Verification items for the finished model (mm, model axes). Round coordinates to 2 decimals unless told otherwise and drop trailing zeros. Order: outer loops, then holes, each group sorted by start corner. A loop starts at its lowest first (then second) coordinate and runs counter-clockwise, first axis right, second up. Notation, with made-up numbers: M 76.5,-8.5 L 121.5,-8.5 A17 cw 121.5,6.5 Z; hole C 83.5,50.25 d2. An arc over 180 degrees is marked long. Use one line per item in the form item = value. Start each with the question number.
Item 1: Cross-section at A-A on x = -7. Enter the section's corners in (y, z).
Item 2: Go/stop test with flat-tipped pins: pin 1 Ø0.6 at (x, z) = (-41, 1.5) entering from +Y; pin 2 Ø1 at (y, z) = (-16.5, 1) entering from -X. Record where each tip stops, or that it passes through.
Item 3: Thickness scan on probe 1 along X at (y, z) = (-7.75, 1.2); probe 2 along X at (y, z) = (-10.25, 1.7); probe 3 along Y at (x, z) = (-41, 1.05). Record the ranges inside material, lowest first. Write a range as [from, to].
Item 4: Cross-section at B-B on x = -35. Enter the section's corners in (y, z).
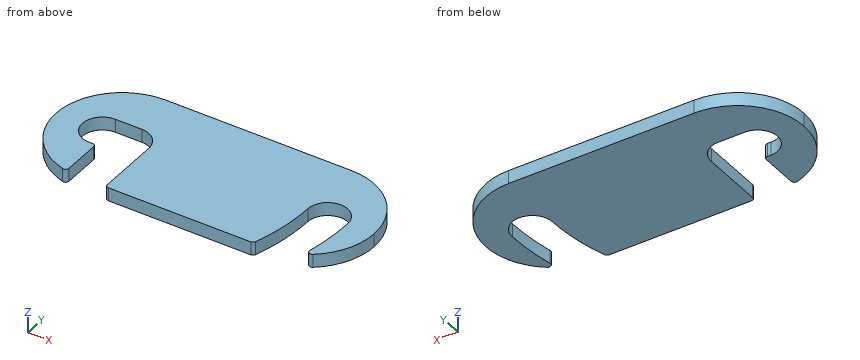
from build123d import *

# Parameters (mm, degrees)
SZKIC1_W                    = 48
SZKIC1_H                    = 20
SZKIC1_R                    = 3
DODANIE_WYCI_GNI_CIE2_DEPTH = 2
ZAOKR_GLENIE3_R             = 10
WYTNIJ_WYCI_GNI_CIE1_DEPTH  = 53.038447325
ZAOKR_GLENIE1_R             = 3
ZAOKR_GLENIE2_R             = 0.5


with BuildPart() as part:
    # Szkic1 → Dodanie-wyciągnięcie2 (new body)
    with BuildSketch(Plane.XY):
        with Locations((-24, -10)):
            Rectangle(SZKIC1_W, SZKIC1_H)
        with Locations((-7, -10)):
            Circle(SZKIC1_R, mode=Mode.SUBTRACT)
        with Locations((-41, -10)):
            Circle(SZKIC1_R, mode=Mode.SUBTRACT)
    extrude(amount=DODANIE_WYCI_GNI_CIE2_DEPTH)

    # Zaokrąglenie3
    zaokr_glenie3_edges = [part.edges().sort_by_distance(p)[0] for p in [
        (0, 0, 1),
        (0, -20, 1),
        (-48, -20, 1),
        (-48, 0, 1),
    ]]
    fillet(zaokr_glenie3_edges, radius=ZAOKR_GLENIE3_R - 0.0001)  # a hair under: the kernel refuses the full size

    # Szkic2 → Wytnij-wyciągnięcie1 (cut, through all)
    with BuildSketch(Plane.XY.offset(2)):
        with BuildLine():
            Line((-10, -10), (-4, -10))
            ThreePointArc((-4, -10), (-4.345859909, -15.047178833), (-5.376973739, -20))
            Line((-5.376973739, -20), (-11.657198498, -20))
            ThreePointArc((-11.657198498, -20), (-10.417105708, -15.068192648), (-10, -10))
        make_face()
        Polygon((-41, -10), (-41, -13), (-40, -13), (-40, -20), (-34, -20), (-34, -17.5), (-34, -7), (-41, -7), align=None)
    extrude(amount=-WYTNIJ_WYCI_GNI_CIE1_DEPTH, mode=Mode.SUBTRACT)

    # Zaokrąglenie1
    zaokr_glenie1_edges = [part.edges().sort_by_distance(p)[0] for p in [
        (-34, -7, 1),
    ]]
    fillet(zaokr_glenie1_edges, radius=ZAOKR_GLENIE1_R)

    # Zaokrąglenie2
    zaokr_glenie2_edges = [part.edges().sort_by_distance(p)[0] for p in [
        (-40, -19.797977321, 1),
        (-5.032269828, -18.678847057, 1),
        (-34, -20, 1),
        (-40, -13, 1),
        (-11.657198498, -20, 1),
    ]]
    fillet(zaokr_glenie2_edges, radius=ZAOKR_GLENIE2_R)


solid = part.part
Output values:
q1.outline = M -7,0 L -0.46,0 L -0.46,2 L -7,2 Z
q2.pin_1 = -0.37
q2.pin_2 = -46
q3.probe_1 = [-47.74, -42.98], [-35.02, -8.98], [-5.02, -0.26]
q3.probe_2 = [-48, -43.99], [-34, -10], [-4, 0]
q3.probe_3 = [-19.54, -13], [-7, -0.46]
q4.outline = M -7.76,0 L 0,0 L 0,2 L -7.76,2 Z
